```python
from build123d import *

# Parameters (mm, degrees)
BOSS_EXTRUDE1_DEPTH = 10
BOSS_EXTRUDE2_DEPTH = 20
SKETCH3_W           = 20
SKETCH3_H           = 10
SKETCH3_W_2         = 15
BOSS_EXTRUDE3_DEPTH = 48.687175822
SKETCH4_R           = 2
SKETCH4_R_2         = 2.5
BOSS_EXTRUDE4_DEPTH = 10
CUT_EXTRUDE1_START  = -4.165511
CUT_EXTRUDE1_DEPTH  = 4.165511
SKETCH8_R           = 45
SKETCH8_R_2         = 36
CUT_EXTRUDE2_DEPTH  = 4.465511


with BuildPart() as part:
    # Sketch1 → Boss-Extrude1 (new body)
    with BuildSketch(Plane(origin=(0, 0, 0), x_dir=(0, 0, -1), z_dir=(1, 0, 0))):
        with BuildLine():
            Line((-47.5, 0), (-27.5, 0))
            ThreePointArc((-27.5, 0), (0, 27.5), (27.5, 0))
            Line((27.5, 0), (47.5, 0))
            ThreePointArc((47.5, 0), (0, 47.5), (-47.5, 0))
        make_face()
    extrude(amount=BOSS_EXTRUDE1_DEPTH)

    # Sketch2 → Boss-Extrude2 (add)
    with BuildSketch(Plane(origin=(10, 0, 0), x_dir=(0, 0, -1), z_dir=(1, 0, 0))):
        with BuildLine():
            Line((-47.5, 0), (-37.5, 0))
            ThreePointArc((-37.5, 0), (0, 37.5), (37.5, 0))
            Line((37.5, 0), (47.5, 0))
            ThreePointArc((47.5, 0), (0, 47.5), (-47.5, 0))
        make_face()
    extrude(amount=BOSS_EXTRUDE2_DEPTH)

    # Sketch3 → Boss-Extrude3 (add)
    with BuildSketch(Plane.XZ):
        with Locations((20, 42.5)):
            Rectangle(SKETCH3_W, SKETCH3_H)
        with Locations((22.5, -42.5)):
            Rectangle(SKETCH3_W_2, SKETCH3_H)
    extrude(amount=BOSS_EXTRUDE3_DEPTH)

    # Sketch4 → Boss-Extrude4 (add)
    with BuildSketch(Plane(origin=(30, 0, 0), x_dir=(0, 0, -1), z_dir=(1, 0, 0))):
        with BuildLine():
            Line((62.5, -48.687175822), (37.5, -48.687175822))
            Line((37.5, -48.687175822), (37.5, 0))
            ThreePointArc((37.5, 0), (0, 37.5), (-37.5, 0))
            Line((-37.5, 0), (-37.5, -48.687175822))
            Line((-37.5, -48.687175822), (-62.5, -48.687175822))
            Line((-62.5, -48.687175822), (-62.5, 0))
            ThreePointArc((-62.5, 0), (0, 62.5), (62.5, 0))
            Line((62.5, 0), (62.5, -48.687175822))
        make_face()
        with Locations((-55, 0)):
            Circle(SKETCH4_R, mode=Mode.SUBTRACT)
        with Locations((0, 55)):
            Circle(SKETCH4_R_2, mode=Mode.SUBTRACT)
        with Locations((-55, -30)):
            Circle(SKETCH4_R, mode=Mode.SUBTRACT)
        with Locations(Location((55, -30, 0), (0, 0, 180))):
            Circle(SKETCH4_R, mode=Mode.SUBTRACT)
        with Locations(Location((55, 0, 0), (0, 0, 180))):
            Circle(SKETCH4_R, mode=Mode.SUBTRACT)
    extrude(amount=BOSS_EXTRUDE4_DEPTH)

    # Sketch7 → Cut-Extrude1 (cut)
    with BuildSketch(Plane(origin=(10, 0, 0), x_dir=(0, 0, -1), z_dir=(1, 0, 0)).offset(CUT_EXTRUDE1_START)):
        with BuildLine():
            Line((27.5, 0), (37.5, 0))
            ThreePointArc((37.5, 0), (0, 37.5), (-37.5, 0))
            Line((-37.5, 0), (-27.5, 0))
            ThreePointArc((-27.5, 0), (0, 27.5), (27.5, 0))
        make_face()
    extrude(amount=CUT_EXTRUDE1_DEPTH, mode=Mode.SUBTRACT)

    # Sketch8 → Cut-Extrude2 (cut)
    with BuildSketch(Plane.ZY.offset(-40)):
        Circle(SKETCH8_R)
        Circle(SKETCH8_R_2, mode=Mode.SUBTRACT)
    extrude(amount=CUT_EXTRUDE2_DEPTH, mode=Mode.SUBTRACT)


solid = part.part
```
Source: CAD feature listing. Evaluate the final solid. Frame: model axes, mm. A direction names the side the tool comes from. Give positions to 0.01 mm unless a question says otherwise; leave off trailing zeros. Loops run counter-clockwise (first coordinate to the right, second up) from the corner with the lowest first, then second, coordinate; pieces in that order, holes last. Notation, with made-up numbers: (80, 78.5) -> (114, 78.5) arc R19 ccw to (114, 104.5) -> close; hole circle Ø3 at (79.25, 85.25). An arc over 180 degrees is marked (long way). Put each result on its own line as item: value. Start each with the question number.
1) Material intervals for probe 1 along Z at (x, y) = (27.5, -40.5); probe 2 along Y at (x, z) = (37.8, 0); probe 3 along Y at (x, z) = (37, 55), sorted ascending.
2) Reachability of faces 5 (the face through (14.79, 47.49, -1.04)), 6 (the face through (27, -25, -37.5)), 7 (the face through (20.48, 37.49, -0.82)) from +Z, -Z, +X, -X, +Y, -Y: full face, straight path, thin tool, end or side. Return the list, or none.
3) Cut plane D-D (y = 25). Return loops of the section in (x, z).
4) Contact query for flat-ended pins moving along their axis: P1, Ø8, axis at x = 16, z = -26, coming from the +Y side; P2, Ø1, axis at x = 34.5, y = 39, coming from the +Z side; P3, Ø5, axis at x = 19.5, y = 7, coming from the +Z side; P4, Ø8, axis at y = 13, z = -40.5, coming from the +X side. Output: stop coordinate, or through.
5) Draft query along Y for faces 1 (the face through (28, -48.687, 47)), 2 (the face through (35, -28, -55)), 3 (the face through (35.534, 39, 0)), 4 (the face through (10, -24, 42)). Return one class per face: released by +Y, released by -Y, zero draft, split by the parting line, or undercut.
6) Cut plane B-B (z = 0). Return loops of the section in (x, y).
7) Cut plane A-A (y = -30). Return loops of the section in (x, z).
8) Cut plane C-C (z = -55). Return loops of the section in (x, y), then the cut area to 3 significant figures.
Results are:
1. probe 1: z = -47.5 to -37.5, 37.5 to 47.5
1. probe 2: y = 45 to 52.5, 57.5 to 62.5
1. probe 3: y = -48.69 to -32, -28 to -2, 2 to 29.69
2. face 5: -X, +Y
2. face 6: +X, -X, -Y
2. face 7: +X, -Y
3. outline: (0, -40.39) -> (30, -40.39) -> (30, -57.28) -> (40, -57.28) -> (40, -37.42) -> (35.53, -37.42) -> (35.53, -27.95) -> (5.83, -27.95) -> (5.83, -11.46) -> (0, -11.46) -> close; (0, 11.46) -> (5.83, 11.46) -> (5.83, 27.95) -> (35.53, 27.95) -> (35.53, 37.42) -> (40, 37.42) -> (40, 57.28) -> (30, 57.28) -> (30, 40.39) -> (0, 40.39) -> close
4. P1: stops at y = 42.1
4. P2: stops at z = 49.23
4. P3: stops at z = 47.29
4. P4: stops at x = 40
5. face 1: released by -Y
5. face 2: undercut
5. face 3: undercut
5. face 4: zero draft
6. outline: (0, 27.5) -> (5.83, 27.5) -> (5.83, 37.5) -> (35.53, 37.5) -> (35.53, 45) -> (40, 45) -> (40, 52.5) -> (30, 52.5) -> (30, 47.5) -> (0, 47.5) -> close; (30, 57.5) -> (40, 57.5) -> (40, 62.5) -> (30, 62.5) -> close
7. outline: (10, 37.5) -> (40, 37.5) -> (40, 53) -> (30, 53) -> (30, 47.5) -> (10, 47.5) -> close; (15, -47.5) -> (30, -47.5) -> (30, -53) -> (40, -53) -> (40, -37.5) -> (15, -37.5) -> close; (30, -62.5) -> (40, -62.5) -> (40, -57) -> (30, -57) -> close; (30, 57) -> (40, 57) -> (40, 62.5) -> (30, 62.5) -> close
8. outline: (30, -48.69) -> (40, -48.69) -> (40, -32) -> (30, -32) -> close; (30, -28) -> (40, -28) -> (40, -2) -> (30, -2) -> close; (30, 2) -> (40, 2) -> (40, 29.69) -> (30, 29.69) -> close
8. area: 704 mm2
